CAD build for the part. Positions are in the model's coordinates, mm. Face numbers are marked on the shaded views. A direction names the side the tool comes from. Give positions to 0.01 mm unless a question says otherwise; leave off trailing zeros. Write each loop counter-clockwise with the first axis right and the second up, starting at its lowest first coordinate (ties: lowest second). Pieces come first, ordered by that corner, then holes. Notation, with made-up numbers: (42.5, -29.5) - (69.5, -29.5) arc R31 cw to (69.5, 8.5) - close; hole circle Ø11 at (-37.75, -32). An arc over 180 degrees is marked (long way). Put each result on its own line as item: value. Start each with the question number.
1. Cut at B-B on y = 0. List the corners of the cut face in (x, z).
2. Cut at A-A on z = 23. List the corners of the cut face in (x, y), and give its area (3 significant figures).
3. Cut at C-C on x = -23.5. List the corners of the cut face in (y, z), and give its area (3 significant figures).
4. Tool access for the marked faces 5, 6, 7 and 8: list every direction of +Z, -Z, +X, -X, +Y, -Y with a clear straight run to the whole face (end or side of a thin tool).
5. Wall check: line 1 (Y direction, x = 0, z = 29.5); line 2 (Z direction, x = -1.5, y = 200.5); line 3 (Z direction, x = -1, y = 194). Give the ranges that are in metal, low to high.
6. Cut at D-D on y = 61. List the corners of the cut face in (x, z), and give its area (3 significant figures).
7. Mould opens along Z. For the marked faces 1, 2, 3 and 4 say: +Z half, -Z half, draft (parallel to the pull), parting line (faces both ways), or undercut.
8. Drop flat-ended pins along their axis: pin 1 (12 mm diameter, centred on x = 10, y = 157.5, fed in from -Z); pin 2 (3 mm diameter, centred on x = 11.5, z = 13.5, fed in from +Y); pin 3 (5 mm diameter, centred on x = -23, y = 136, fed in from -Z). Give the stop position or say it passes through.
from build123d import *

# Parameters (mm, degrees)
BOSS_EXTRUDE1_DEPTH      = 45
CUT_EXTRUDE2_DEPTH       = 36
CUT_EXTRUDE2_DEPTH_BACK  = 36
CUT_EXTRUDE3_DEPTH       = 28
SKETCH6_R                = 4.5
SKETCH6_R_2              = 2.5
CUT_EXTRUDE4_DEPTH       = 29
CUT_EXTRUDE4_DEPTH_BACK  = 18
CUT_EXTRUDE6_DEPTH       = 10
SKETCH12_W               = 33
SKETCH12_H               = 40
CUT_EXTRUDE9_DEPTH       = 9
CUT_EXTRUDE9_DEPTH_BACK  = 9
SKETCH13_W               = 31
SKETCH13_H               = 35
CUT_EXTRUDE10_DEPTH      = 36
CUT_EXTRUDE10_DEPTH_BACK = 36
SKETCH14_R               = 2
CUT_EXTRUDE13_DEPTH      = 46
CUT_EXTRUDE13_DEPTH_BACK = 9
SKETCH15_R               = 2.5
CUT_EXTRUDE14_DEPTH      = 16.676509358


with BuildPart() as part:
    # Sketch1 → Boss-Extrude1 (new body)
    with BuildSketch(Plane.XY):
        with BuildLine():
            Line((-12.137605226, 40.130176139), (-28.41462727, 172.695882476))
            ThreePointArc((-28.41462727, 172.695882476), (-25.871526221, 185.155210183), (-16.331642516, 193.563112938))
            ThreePointArc((-16.331642516, 193.563112938), (-13.372104724, 195.395277041), (-12.437153877, 198.748120036))
            ThreePointArc((-12.437153877, 198.748120036), (0, 212.5), (12.437153877, 198.748120036))
            ThreePointArc((12.437153877, 198.748120036), (13.372104724, 195.395277041), (16.331642516, 193.563112938))
            ThreePointArc((16.331642516, 193.563112938), (25.871526221, 185.155210183), (28.41462727, 172.695882476))
            Line((28.41462727, 172.695882476), (12.137605226, 40.130176139))
            ThreePointArc((12.137605226, 40.130176139), (13.235334505, 34.563989878), (17.184596043, 30.490812695))
            ThreePointArc((17.184596043, 30.490812695), (0, -35), (-17.184596043, 30.490812695))
            ThreePointArc((-17.184596043, 30.490812695), (-13.235334505, 34.563989878), (-12.137605226, 40.130176139))
        make_face()
    extrude(amount=BOSS_EXTRUDE1_DEPTH)

    # Sketch4 → Cut-Extrude2 (cut, two sides)
    with BuildSketch(Plane(origin=(0, 0, 0), x_dir=(0, 0, -1), z_dir=(1, 0, 0))) as cut_extrude2_sk:
        Polygon((-45, 196.155616487), (-33, 30.490812695), (-33, -35), (-45, -35), align=None)
        Polygon((-12, -35), (0, -35), (0, 196.155616487), (-12, 30.490812695), align=None)
    extrude(amount=CUT_EXTRUDE2_DEPTH, mode=Mode.SUBTRACT)
    extrude(cut_extrude2_sk.sketch, amount=-CUT_EXTRUDE2_DEPTH_BACK, mode=Mode.SUBTRACT)

    # Sketch5 → Cut-Extrude3 (cut)
    with BuildSketch(Plane.XY):
        Polygon((16.97, -20.5), (-16.97, -20.5), (-20.5, -16.97), (-20.5, 16.97), (-16.97, 20.5), (16.97, 20.5), (20.5, 16.97), (20.5, -16.97), align=None)
    extrude(amount=CUT_EXTRUDE3_DEPTH, mode=Mode.SUBTRACT)

    # Sketch6 → Cut-Extrude4 (cut, two sides)
    with BuildSketch(Plane(origin=(0, 0, 28), x_dir=(-1, 0, 0), z_dir=(0, 0, -1))) as cut_extrude4_sk:
        Circle(SKETCH6_R)
        with Locations((-16.257359313, 16.257359313)):
            Circle(SKETCH6_R_2)
        with Locations((16.260126266, 16.260126266)):
            Circle(SKETCH6_R_2)
        with Locations((-16.260126266, -16.260126266)):
            Circle(SKETCH6_R_2)
        with Locations((16.260126266, -16.260126266)):
            Circle(SKETCH6_R_2)
    extrude(amount=CUT_EXTRUDE4_DEPTH, mode=Mode.SUBTRACT)
    extrude(cut_extrude4_sk.sketch, amount=-CUT_EXTRUDE4_DEPTH_BACK, mode=Mode.SUBTRACT)

    # Sketch8 → Cut-Extrude6 (cut, along a direction that is not the sketch's normal)
    with BuildSketch(Plane(origin=(0, 1.023835067, 14.134452964), x_dir=(-1, 0, 0), z_dir=(0, -0.072246136, -0.997386834))):
        with BuildLine():
            Line((-2.88453501, 56.792957469), (-14.82487519, 154.294010847))
            ThreePointArc((-14.82487519, 154.294010847), (0.17238227, 165.145626965), (15.16963973, 154.294010847))
            Line((15.16963973, 154.294010847), (3.214085595, 56.668725114))
            ThreePointArc((3.214085595, 56.668725114), (0.089957546, 53.058005434), (-2.88453501, 56.792957469))
        make_face()
    extrude(amount=-CUT_EXTRUDE6_DEPTH, dir=(0, 0.072246136, -0.997386834), mode=Mode.SUBTRACT)

    # Sketch12 → Cut-Extrude9 (cut, two sides)
    with BuildSketch(Plane(origin=(0, 0, 0), x_dir=(0, 0, -1), z_dir=(1, 0, 0))) as cut_extrude9_sk:
        with Locations((-32.176509358, 158.99066374)):
            Rectangle(SKETCH12_W, SKETCH12_H)
    extrude(amount=CUT_EXTRUDE9_DEPTH, mode=Mode.SUBTRACT)
    extrude(cut_extrude9_sk.sketch, amount=-CUT_EXTRUDE9_DEPTH_BACK, mode=Mode.SUBTRACT)

    # Sketch13 → Cut-Extrude10 (cut, two sides)
    with BuildSketch(Plane(origin=(0, 0, 0), x_dir=(0, 0, -1), z_dir=(1, 0, 0))) as cut_extrude10_sk:
        with Locations((-22.5, 195)):
            Rectangle(SKETCH13_W, SKETCH13_H)
    extrude(amount=CUT_EXTRUDE10_DEPTH, mode=Mode.SUBTRACT)
    extrude(cut_extrude10_sk.sketch, amount=-CUT_EXTRUDE10_DEPTH_BACK, mode=Mode.SUBTRACT)

    # Sketch14 → Cut-Extrude13 (cut, two sides)
    with BuildSketch(Plane.XY) as cut_extrude13_sk:
        with Locations((0, 203.896404583)):
            Circle(SKETCH14_R)
    extrude(amount=CUT_EXTRUDE13_DEPTH, mode=Mode.SUBTRACT)
    extrude(cut_extrude13_sk.sketch, amount=-CUT_EXTRUDE13_DEPTH_BACK, mode=Mode.SUBTRACT)

    # Sketch15 → Cut-Extrude14 (cut, through all)
    with BuildSketch(Plane.XY.offset(15.676509358)):
        with Locations((0, 167.5)):
            Circle(SKETCH15_R)
    extrude(amount=-CUT_EXTRUDE14_DEPTH, mode=Mode.SUBTRACT)


solid = part.part
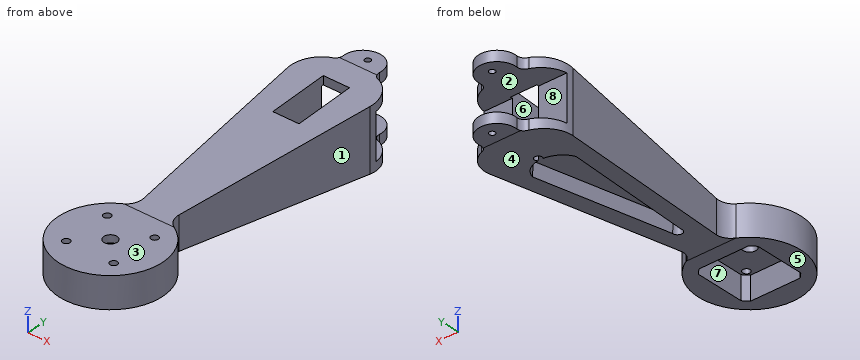
Report:
1. outline: (-35, 12) - (-20.5, 12) - (-20.5, 28) - (-4.5, 28) - (-4.5, 33) - (-35, 33) - close; (4.5, 28) - (20.5, 28) - (20.5, 12) - (35, 12) - (35, 33) - (4.5, 33) - close
2. outline: (-28.42, 177.5) arc R20 ccw to (-28.41, 172.7) - (-12.14, 40.13) arc R10 cw to (-17.18, 30.49) arc R35 ccw (long way) to (17.18, 30.49) arc R10 cw to (12.14, 40.13) - (28.41, 172.7) arc R20 ccw to (28.42, 177.5) - (9, 177.5) - (9, 138.99) - (-9, 138.99) - (-9, 177.5) - close; hole (-20.5, -16.97) - (-16.97, -20.5) - (16.97, -20.5) - (20.5, -16.97) - (20.5, 16.97) - (16.97, 20.5) - (-16.97, 20.5) - (-20.5, 16.97) - close
2. area: 7,300 mm²
3. outline: (-25.94, 12) - (25.94, 12) - (25.94, 33) - (-25.94, 33) - close; (132.67, 4.6) - (188.43, 0.56) - (188.43, 7) - (177.5, 7) - (177.5, 38) - (188.43, 38) - (188.43, 44.44) - (132.67, 40.4) - close
3. area: 2,970 mm²
4. face 5: -Z, +X, -X, -Y
4. face 6: +Z
4. face 7: -Z
4. face 8: +X, -X, +Y
5. line 1: y = -35 to -4.5, 4.5 to 138.99
5. line 2: z = 0 to 7, 38 to 45
5. line 3: z = 0.16 to 7, 38 to 44.84
6. outline: (-14.7, 9.79) - (-3.64, 9.79) - (-3.73, 19.71) - (3.38, 19.71) - (3.29, 9.79) - (14.7, 9.79) - (14.7, 35.21) - (-14.7, 35.21) - close
6. area: 678 mm²
7. face 1: draft
7. face 2: undercut
7. face 3: +Z half
7. face 4: -Z half
8. pin 1: stops at z = 2.37
8. pin 2: stops at y = 177.5
8. pin 3: stops at z = 4.18
